Autodesk Inventor part; units mm, degrees
ref_plane "YZ Plane" through (0, 0, 0) normal (1, 0, 0) x (0, 1, 0)
ref_plane "XZ Plane" through (0, 0, 0) normal (0, 1, 0) x (-1, 0, 0)
ref_plane "XY Plane" through (0, 0, 0) normal (0, 0, 1) x (1, 0, 0)
sketch "草图1" plane through (0, 0, 0) normal (0, 0, 1) x (1, 0, 0)
  circle A0 centre (0, 0) radius 60
  dimension "d0" = 120
extrude "拉伸1" add sketch "草图1" along normal blind 100
shell "抽壳1" thickness 10 removed faces 1 at (20.3445, -12.2, 100)
sketch "草图2" plane through (0, 0, 0) normal (0, 1, 0) x (-1, 0, 0)
  point P0 (0, 0)
  point P1 (0, 80)
  dimension "d4" = 80
hole "孔1" at (0, 0, 80) direction (0, -1, 0) diameter 10 end through all both
properties part number "活塞"
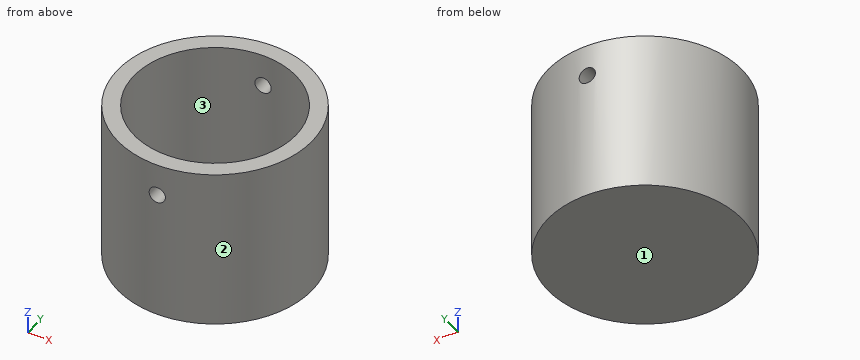
Input: part model. Units: mm. Frame: model coordinates. Face numbers are marked on the shaded views. Give positions to 0.01 mm unless a question says otherwise; leave off trailing zeros. Write each loop counter-clockwise with the first axis right and the second up, starting at its lowest first coordinate (ties: lowest second). Pieces come first, ordered by that corner, then holes. Notation, with made-up numbers: M 31,52 L 70,52 A22 ccw 70,71 Z; hole C 48.25,35.25 d5. An arc over 180 degrees is marked long. Write item = value, one per line. Start each with the question number.
1) Cut plane A-A on x = 0. Return the cut outline in (y, z).
2) Material intervals for line 1 along Z through (x, y) = (0, -55); line 2 along Y through (x, z) = (0, 50); line 3 along Z through (x, y) = (15.5, -37.5), sorted ascending. Write a range as [from, to].
3) Draft query along Y for the marked faces 1, 2 and 3. Return one class per face: +Y half, -Y half, draft (parallel to the pull), parting line (faces both ways), or undercut.
4) Cut plane C-C on z = 80. Return the cut outline in (x, y), then the cut area to 3 significant figures.
5) Cut plane D-D on x = 30.5. Return the cut outline in (y, z).
6) Cut plane B-B on y = 0. Return the cut outline in (x, z), then the cut area to 3 significant figures.
7) First-contact query: pin 1 Ø10 at (y, z) = (9, 33.5) entering from -X; pin 2 Ø10 at (y, z) = (41.5, 10.5) entering from +X; pin 3 Ø6 at (x, z) = (0, 80) entering from -Y; pin 4 Ø5 at (x, y) = (19, -4) entering from +Z. Flat tips, straight axial feed; report the tip coordinate or a pass-through.
Solved:
q1.outline = M -60,0 L 60,0 L 60,75 L 50,75 L 50,10 L -50,10 L -50,75 L -60,75 Z; M -60,85 L -50,85 L -50,100 L -60,100 Z; M 50,85 L 60,85 L 60,100 L 50,100 Z
q2.line_1 = [0, 75], [85, 100]
q2.line_2 = [-60, -50], [50, 60]
q2.line_3 = [0, 10]
q3.face_1 = draft
q3.face_2 = parting line
q3.face_3 = undercut
q4.outline = M -5,-59.79 L -5,-49.75 A50 cw -5,49.75 L -5,59.79 A60 ccw Z; M 5,-59.79 A60 ccw 5,59.79 L 5,49.75 A50 cw 5,-49.75 Z
q4.area = 3,260 mm2
q5.outline = M -51.67,0 L 51.67,0 L 51.67,100 L 39.62,100 L 39.62,10 L -39.62,10 L -39.62,100 L -51.67,100 Z
q6.outline = M -60,0 L 60,0 L 60,100 L 50,100 L 50,10 L -50,10 L -50,100 L -60,100 Z
q6.area = 3,000 mm2
q7.pin_1 = -59.87
q7.pin_2 = 47.62
q7.pin_3 = through
q7.pin_4 = 10
